Answer from the drawing. Dimensions are ordinates in mm from the lowest x, y and z of the part. Coordinates: 2 decimals unless noted, no trailing zeros. Write each loop counter-clockwise with the first axis right and the second up, starting at its lowest first coordinate (ties: lowest second). Pieces come first, ordered by that corner, then holes.
(1) The part is cut by section C-C, the plane x = 84. Determine the outline of the cut face in (y, z) (1 decimal).
(2) Given pin 1 (4 mm diameter, centred on x = 51.5, z = 6, fed in from +Y); pin 2 (4 mm diameter, centred on x = 17.5, z = 8, fed in from -Y); pin 3 (9 mm diameter, centred on x = 62.5, y = 5.5, fed in from -Z), each flat-ended and moving along its own axis, determine where each tip first touches the part or whether it passes through.
(3) The part is cut by section A-A, the plane y = 62.5. Determine the outline of the cut face in (x, z), and give its area (3 significant figures).
(4) The part is cut by section D-D, the plane z = 7.5. State how many separate pieces and enclosed holes the cut face has, and give its area (3 significant figures).
(5) Straight lines are drawn through the part: line 1 along Y through (x, z) = (62.5, 8.9); line 2 along X through (y, z) = (14.5, 5.5) (1 decimal); line 3 along Z through (x, y) = (7.5, 58). For each, find the intervals that lie inside material, in ascending order.
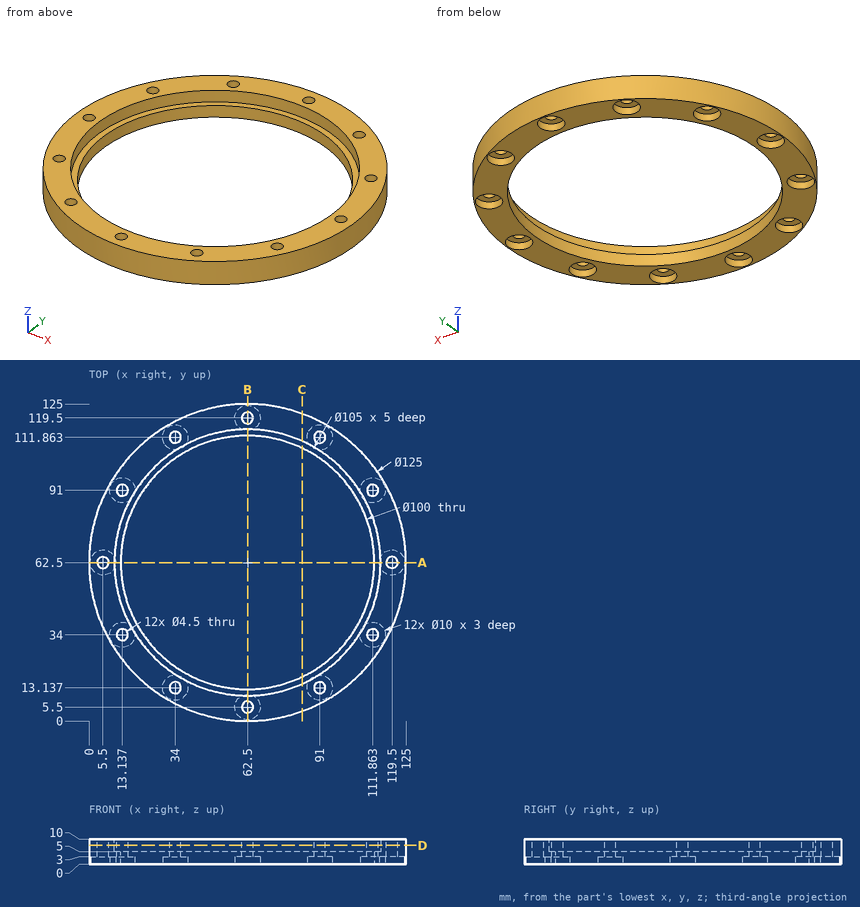
Computed:
1. outline: (3.8, 0) - (17.4, 0) - (17.4, 5) - (14.6, 5) - (14.6, 10) - (3.8, 10) - close; (107.6, 0) - (121.2, 0) - (121.2, 10) - (110.4, 10) - (110.4, 5) - (107.6, 5) - close
2. pin 1: stops at y = 124.35
2. pin 2: stops at y = 17.14
2. pin 3: stops at z = 3
3. outline: (0, 0) - (0.5, 0) - (0.5, 3) - (3.25, 3) - (3.25, 10) - (0, 10) - close; (7.75, 3) - (10.5, 3) - (10.5, 0) - (12.5, 0) - (12.5, 5) - (10, 5) - (10, 10) - (7.75, 10) - close; (112.5, 0) - (114.5, 0) - (114.5, 3) - (117.25, 3) - (117.25, 10) - (115, 10) - (115, 5) - (112.5, 5) - close; (121.75, 3) - (124.5, 3) - (124.5, 0) - (125, 0) - (125, 10) - (121.75, 10) - close
3. area: 102 mm2
4. separate pieces: 1
4. enclosed holes: 13
4. area: 3,420 mm2
5. line 1: y = 0 to 3.25, 7.75 to 10, 115 to 117.25, 121.75 to 125
5. line 2: x = 22.5 to 32.2, 35.8 to 41.2, 83.8 to 89.2, 92.8 to 102.5
5. line 3: z = 3 to 10
